Autodesk Inventor part; units mm, degrees
ref_plane "YZ Plane" through (0, 0, 0) normal (1, 0, 0) x (0, 1, 0)
ref_plane "XZ Plane" through (0, 0, 0) normal (0, 1, 0) x (-1, 0, 0)
ref_plane "XY Plane" through (0, 0, 0) normal (0, 0, 1) x (1, 0, 0)
sketch "Sketch1" plane through (0, 0, 0) normal (0, 1, 0) x (-1, 0, 0)
  line L0 (-14, -58.75) -> (-19, -58.75)
  line L1 (-35.25, 21.625) -> (35.25, 21.625)
  line L2 (-35.25, 21.625) -> (35.25, 21.625) construction
  line L3 (35.25, 21.625) -> (25.25, 21.625)
  line L4 (-35.25, 21.625) -> (35.25, 21.625)
  line L5 (35.25, 21.625) -> (35.25, -69.875)
  line L6 (35.25, -69.875) -> (-35.25, -69.875)
  line L7 (-35.25, -69.875) -> (-35.25, 21.625)
  line L8 (-35.25, 21.625) -> (-35.25, 11.625)
  line L9 (-35.25, 11.625) -> (-25.25, 11.625)
  circle A0 centre (-25.25, 11.625) radius 3.5
  line L10 (35.25, 21.625) -> (25.25, 21.625)
  line L11 (25.25, 21.625) -> (25.25, 11.625)
  circle A1 centre (25.25, 11.625) radius 3.5
  line L12 (35.25, -69.875) -> (25.25, -69.875)
  line L13 (25.25, -69.875) -> (25.25, -59.875)
  circle A2 centre (25.25, -59.875) radius 3.5
  line L14 (-35.25, -69.875) -> (-25.25, -69.875)
  line L15 (-25.25, -69.875) -> (-25.25, -59.875)
  circle A3 centre (-25.25, -59.875) radius 3.5
  line L16 (-25.25, 11.625) -> (-25.25, -18.375)
  line L17 (25.25, -59.875) -> (25.25, -29.875)
  circle A4 centre (-25.25, -18.375) radius 2.5
  circle A5 centre (25.25, -29.875) radius 2.5
  point P0 (0, 0)
  dimension "d6" = 5
  dimension "d9" = 70.5
  dimension "d41" = 70.5
  dimension "d42" = 91.5
  dimension "d43" = 10
  dimension "d44" = 10
  dimension "d45" = 7
  dimension "d46" = 10
  dimension "d47" = 10
  dimension "d48" = 90
  dimension "d50" = 7
  dimension "d51" = 10
  dimension "d52" = 10
  dimension "d53" = 7
  dimension "d54" = 10
  dimension "d55" = 10
  dimension "d56" = 7
  dimension "d60" = 30
  dimension "d61" = 30
  dimension "d62" = 5
  dimension "d63" = 5
extrude "Extrusion1" add sketch "Sketch1" along normal blind 6
properties part number "m"
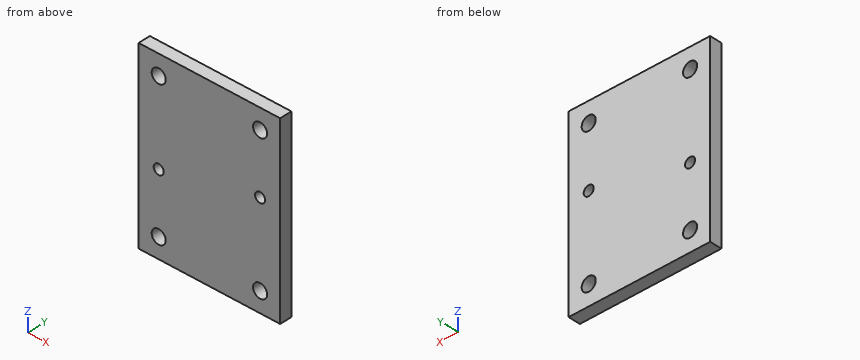
Read the model definition and answer for the solid it produces. Units are mm, in the model's axes. Give positions to 0.01 mm unless a question says otherwise; leave off trailing zeros. Loops run counter-clockwise (first coordinate to the right, second up) from the corner with the lowest first, then second, coordinate; pieces in that order, holes last. Notation, with made-up numbers: M 12.5,72 L 42.5,72 A19 ccw 42.5,82 Z; hole C 72,47 d5. An arc over 180 degrees is marked long. Write each question's results on one line, items separated by ' | '.
1. Straight lines are drawn through the part: line 1 (Z direction, x = 25.25, y = 4.2) (3 decimals); line 2 (X direction, y = 2.3, z = 14); line 3 (X direction, y = 2.1, z = -30). For each, find the intervals that lie inside material, in ascending order. Write a range as [from, to].
Values:
line 1: z = [-69.875, -63.375], [-56.375, -20.875], [-15.875, 8.125], [15.125, 21.625] | line 2: x = [-35.25, -27.82], [-22.68, 22.68], [27.82, 35.25] | line 3: x = [-35.25, -27.75], [-22.75, 35.25]
2. Section B-B on y = 2.15 is taken. Give the vertices of the cut face in (x, z) (3 decimals), plus the area to 3 significant figures.
Values:
outline: M -35.25,-69.875 L 35.25,-69.875 L 35.25,21.625 L -35.25,21.625 Z; hole C -25.25,-59.875 d7; hole C -25.25,11.625 d7; hole C -25.25,-29.875 d5; hole C 25.25,-59.875 d7; hole C 25.25,11.625 d7; hole C 25.25,-18.375 d5 | area: 6,260 mm^2
3. Given pin 1 (9 mm diameter, centred on x = -25.25, z = 11.625, fed in from +Y); pin 2 (5.5 mm diameter, centred on x = 25.25, z = 11.625, fed in from +Y), each flat-ended and moving along its own axis, determine where each tip first touches the part or whether it passes through.
Values:
pin 1: stops at y = 6 | pin 2: passes through
4. Section A-A on x = 25.25 is taken. Give the vertices of the cut face in (y, z) (3 decimals), plus the area to 3 significant figures.
Values:
outline: M 0,-69.875 L 6,-69.875 L 6,-63.375 L 0,-63.375 Z; M 0,-56.375 L 6,-56.375 L 6,-20.875 L 0,-20.875 Z; M 0,-15.875 L 6,-15.875 L 6,8.125 L 0,8.125 Z; M 0,15.125 L 6,15.125 L 6,21.625 L 0,21.625 Z | area: 435 mm^2
